Autodesk Inventor part; units mm, degrees
ref_plane "YZ Plane" through (0, 0, 0) normal (1, 0, 0) x (0, 1, 0)
ref_plane "XZ Plane" through (0, 0, 0) normal (0, 1, 0) x (-1, 0, 0)
ref_plane "XY Plane" through (0, 0, 0) normal (0, 0, 1) x (1, 0, 0)
sketch "Sketch8" plane through (0, 0, 0) normal (0, 0, 1) x (1, 0, 0)
  line L0 (-930, 50) -> (930, 50)
  line L1 (930, 50) -> (930, 0)
  line L2 (930, 0) -> (-930, 0)
  line L3 (-930, 0) -> (-930, 50)
  point P0 (0, 0)
  point P1 (0, 0)
  dimension "d37" = 50
  dimension "d38" = 1860
extrude "Plate5" add sketch "Sketch8" against normal blind 3
sketch "Sketch9" plane through (0, 0, 0) normal (0, 0, 1) x (1, 0, 0)
  line L0 (930, 50) -> (-930, 50)
  line L1 (-784, 50) -> (-780.8, 50)
  line L2 (-780.8, 50) -> (-780.8, 24)
  line L3 (-780.8, 24) -> (-784, 24)
  line L4 (-784, 24) -> (-784, 50)
  line L5 (-930, 50) -> (-930, 0)
  point P0 (0, 0)
  point P1 (-780.8, 50)
  dimension "d42" = 146
  dimension "d43" = 3.2
  dimension "d44" = 26
extrude "Extrusion3" cut sketch "Sketch9" against normal through all
pattern_linear "Rectangular Pattern2" count 6 spacing 500 along (1, 0, 0) of "Extrusion3"
sketch "Sketch10" plane through (0, 0, 0) normal (0, 0, 1) x (1, 0, 0)
  line L0 (930, 50) -> (719.2, 50)
  line L1 (719.2, 50) -> (719.2, 24)
  line L2 (719.2, 24) -> (716, 24)
  line L3 (716, 24) -> (716, 50)
  line L4 (716, 50) -> (219.2, 50)
  line L5 (219.2, 50) -> (219.2, 24)
  line L6 (219.2, 24) -> (216, 24)
  line L7 (216, 24) -> (216, 50)
  line L8 (216, 50) -> (-280.8, 50)
  line L9 (-280.8, 50) -> (-280.8, 24)
  line L10 (-280.8, 24) -> (-284, 24)
  line L11 (-284, 24) -> (-284, 50)
  line L12 (-284, 50) -> (-780.8, 50)
  line L13 (-780.8, 50) -> (-780.8, 24)
  line L14 (-780.8, 24) -> (-784, 24)
  line L15 (-784, 24) -> (-784, 50)
  line L16 (-784, 50) -> (-930, 50)
  line L17 (-930, 50) -> (-930, 0)
  line L18 (-930, 0) -> (930, 0)
  line L19 (930, 0) -> (930, 50)
  circle A0 centre (440, 50) radius 20
  point P0 (0, 0)
  point P1 (420, 50)
  point P2 (460, 50)
  point P3 (50, 50)
  point P4 (90, 50)
  dimension "d50" = 40
  dimension "d52" = 1370
extrude "Extrusion4" cut sketch "Sketch10" against normal through all contours A0 L4 | L4 A0
sketch "Sketch11" plane through (0, 0, 0) normal (0, 0, 1) x (1, 0, 0)
  line L0 (-752.5883, 29.3223) -> (-521.0772, 29.3223) construction
  line L1 (-521.0772, 29.3223) -> (-521.0772, 13.038) construction
  line L2 (-521.0772, 13.038) -> (-752.5883, 13.038) construction
  line L3 (-752.5883, 13.038) -> (-752.5883, 29.3223) construction
  point P0 (0, 0)
mark "Mark1"
equation "\"d41\" = Thickness"
equation "\"BendReliefWidth\" = Thickness"
equation "\"BendReliefDepth\" = 0.5 * Thickness"
equation "\"CornerReliefSize\" = 4 * Thickness"
equation "\"MinimumRemnant\" = 2 * Thickness"
equation "\"TransitionRadius\" = BendRadius"
equation "\"JacobiRadiusSize\" = BendRadius"
equation "\"GapSize\" = Thickness"
properties part number "BSH 033 stringer floor 3" material "09g2s"
Geometry: final body of the model. Coordinates: model frame, mm. Coordinates: 2 decimals unless noted, no trailing zeros. Write each loop counter-clockwise with the first axis right and the second up, starting at its lowest first coordinate (ties: lowest second). Pieces come first, ordered by that corner, then holes. Notation, with made-up numbers: M 6.25,67 L 34.25,67 A24 ccw 34.25,81 Z; hole C 76.25,-23 d2. An arc over 180 degrees is marked long. Use CSV: the item, a comma, the result in double quotes. Start each with the question number.
1. Ray query, probe 1 along X at (y, z) = (27.5, -1.85); probe 2 along X at (y, z) = (47, -2.8); probe 3 along X at (y, z) = (36.5, -1.2). Return the intervals inside material, ascending.
2. Cut plane A-A on y = 42.5. Return the cut outline in (x, z).
3. Cut plane B-B on x = 440. Return the cut outline in (y, z), plus the area to 3 significant figures.
4. First-contact query: P1, Ø1.5, axis at x = -782, z = -1, coming from the +Y side. Flat tip, straight axial feed; report the tip coordinate or a pass-through.
Entries:
1,probe 1,"-930 to -784, -780.8 to -284, -280.8 to 216, 219.2 to 716, 719.2 to 930"
1,probe 2,"-930 to -784, -780.8 to -284, -280.8 to 216, 219.2 to 420.23, 459.77 to 716, 719.2 to 930"
1,probe 3,"-930 to -784, -780.8 to -284, -280.8 to 216, 219.2 to 425.24, 454.76 to 716, 719.2 to 930"
2,outline,"M -930,-3 L -784,-3 L -784,0 L -930,0 Z; M -780.8,-3 L -284,-3 L -284,0 L -780.8,0 Z; M -280.8,-3 L 216,-3 L 216,0 L -280.8,0 Z; M 219.2,-3 L 421.46,-3 L 421.46,0 L 219.2,0 Z; M 458.54,-3 L 716,-3 L 716,0 L 458.54,0 Z; M 719.2,-3 L 930,-3 L 930,0 L 719.2,0 Z"
3,outline,"M 0,-3 L 30,-3 L 30,0 L 0,0 Z"
3,area,"90.0 mm²"
4,P1,"y = 24"
